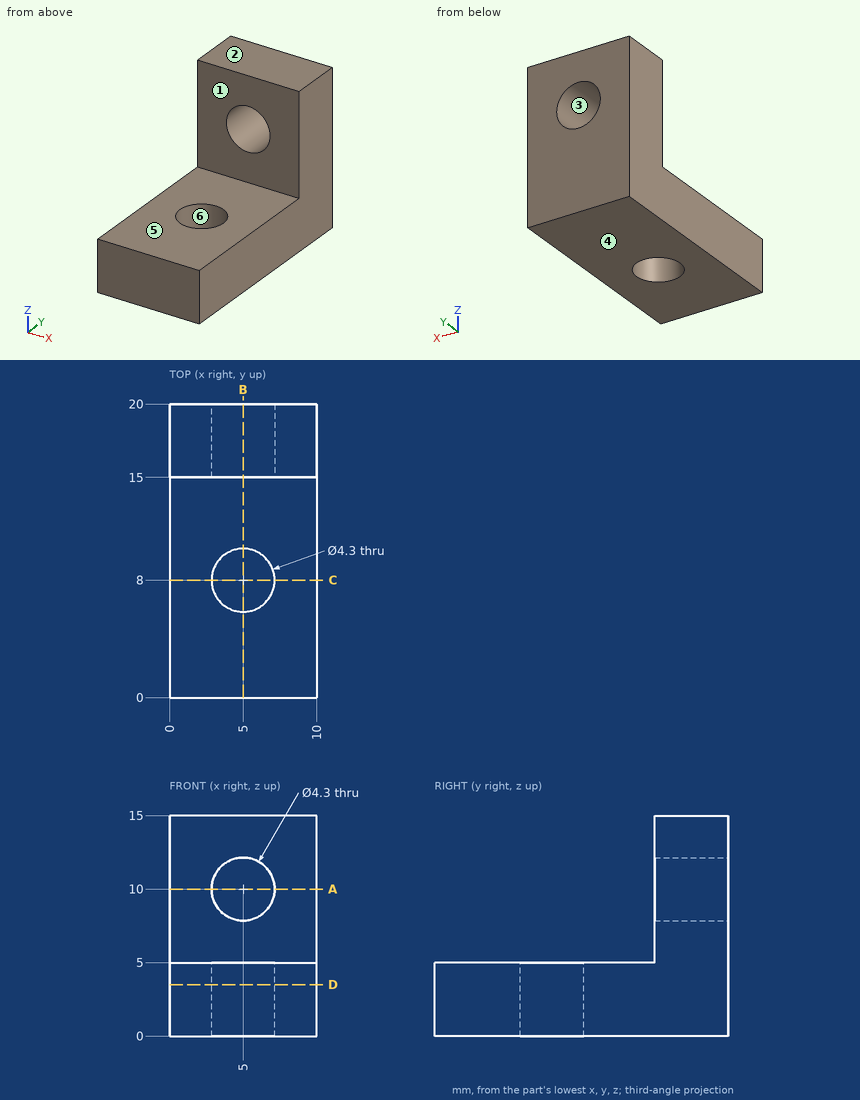
Geometry: see drawing. Coordinates: mm, zero at the bounding-box minimum. A direction names the side the tool comes from. Give positions to 0.01 mm unless a question says otherwise; leave off trailing zeros. Loops run counter-clockwise (first coordinate to the right, second up) from the corner with the lowest first, then second, coordinate; pieces in that order, holes last. Notation, with made-up numbers: M -2,12 L 57,12 A17 ccw 57,27 Z; hole C 63.5,34.5 d2. An arc over 180 degrees is marked long. Use one line per item in the form item = value.
1. Section query C-C, the plane y = 8. Return the cut outline in (x, z), and give its area (3 significant figures).
Numbers:
outline = M 0,0 L 2.85,0 L 2.85,5 L 0,5 Z; M 7.15,0 L 10,0 L 10,5 L 7.15,5 Z
area = 28.5 mm²
2. Section query B-B, the plane x = 5. Return the cut outline in (y, z), and give its area (3 significant figures).
Numbers:
outline = M 0,0 L 5.85,0 L 5.85,5 L 0,5 Z; M 10.15,0 L 20,0 L 20,7.85 L 15,7.85 L 15,5 L 10.15,5 Z; M 15,12.15 L 20,12.15 L 20,15 L 15,15 Z
area = 107 mm²
3. Section query A-A, the plane z = 10. Return the cut outline in (x, y).
Numbers:
outline = M 0,15 L 2.85,15 L 2.85,20 L 0,20 Z; M 7.15,15 L 10,15 L 10,20 L 7.15,20 Z
4. Reachability of the marked faces 1 and 2 from +Z, -Z, +X, -X, +Y, -Y: full face, straight path, thin tool, end or side. Return the list, or none.
Numbers:
face_1 = +Z, +X, -X, -Y
face_2 = +Z, +X, -X, +Y, -Y
5. Pull-direction query (Z, two-part tool) for the marked faces 3, 4, 5 and 6; classes: released by +Z, released by -Z, zero draft, split by the parting line, or undercut.
Numbers:
face_3 = undercut
face_4 = released by -Z
face_5 = released by +Z
face_6 = zero draft
6. Section query D-D, the plane z = 3.5. Return the cut outline in (x, y), and give its area (3 significant figures).
Numbers:
outline = M 0,0 L 10,0 L 10,20 L 0,20 Z; hole C 5,8 d4.3
area = 185 mm²
7. Line query: L1, parallel to Z at x = 5, y = 19; L2, parallel to Y at x = 5, z = 2.4; L3, parallel to X at y = 18.6, z = 10. Output: solid intervals per line, ascending.
Numbers:
L1 = 0 to 7.85, 12.15 to 15
L2 = 0 to 5.85, 10.15 to 20
L3 = 0 to 2.85, 7.15 to 10
8. First-contact query: pin 1 (5 mm diameter, centred on x = 2, y = 3, fed in from +Z); pin 2 (5 mm diameter, centred on x = 5, z = 11.5, fed in from -Y); pin 3 (4 mm diameter, centred on x = 2.5, y = 6.5, fed in from -Z). Flat tips, straight axial feed; report the tip coordinate or a pass-through.
Numbers:
pin_1 = 5
pin_2 = 15
pin_3 = 0
